from build123d import *

# Parameters (mm, degrees)
F3_DEPTH = 46.501
F5_D     = 14
F6_R     = 2
F7_R     = 1
F8_SIZE  = 1
F9_SIZE  = 0.5
F10_R    = 0.4


with BuildPart() as f1:
    # F0 (on Right) → F1 (revolve)
    with BuildSketch(Plane.YZ):
        Polygon((1.5, 26), (0, 26), (0, 16), (46.5, 16), (46.5, 28), (19.5, 28), (19.5, 62.5), (1.5, 62.5), align=None)
    revolve(axis=Axis((0, 26.823761, 0), (0, 1, 0)))

    # F2 (on face) → F3 (cut, through all)
    with BuildSketch(Plane(origin=(0, 46.5, 0), x_dir=(-1, 0, 0), z_dir=(0, 1, 0))):
        with BuildLine():
            ThreePointArc((4, 15.491933), (0, 16), (-4, 15.491933))
            Line((-4, 15.491933), (-4, 12))
            Line((-4, 12), (4, 12))
            Line((4, 12), (4, 15.491933))
        make_face()
        with BuildLine():
            Line((4, 18.4), (-4, 18.4))
            Line((-4, 18.4), (-4, 15.491933))
            ThreePointArc((-4, 15.491933), (0, 16), (4, 15.491933))
            Line((4, 15.491933), (4, 18.4))
        make_face()
    extrude(amount=-F3_DEPTH, mode=Mode.SUBTRACT)

    # F5 (through all)
    with Locations(Plane(origin=(0, 19.5, 0), x_dir=(-1, 0, 0), z_dir=(0, 1, 0))):
        with Locations((-30.052038, 30.052038), (30.052038, 30.052038), (-30.052038, -30.052038), (30.052038, -30.052038)):
            Hole(F5_D / 2)

    # F6
    f6_edges = [f1.edges().sort_by_distance(p)[0] for p in [
        (0, 19.5, -28),
        (0, 46.5, -28),
    ]]
    fillet(f6_edges, radius=F6_R)

    # F7
    f7_edges = [f1.edges().sort_by_distance(p)[0] for p in [
        (0, 19.5, -62.5),
    ]]
    fillet(f7_edges, radius=F7_R)

    # F8
    f8_edges = [f1.edges().sort_by_distance(p)[0] for p in [
        (0, 1.5, -62.5),
    ]]
    chamfer(f8_edges, length=F8_SIZE)

    # F9
    f9_edges = [f1.edges().sort_by_distance(p)[0] for p in [
        (0, 0, -26),
    ]]
    chamfer(f9_edges, length=F9_SIZE)

    # F10
    f10_edges = [f1.edges().sort_by_distance(p)[0] for p in [
        (0, 1.5, -26),
    ]]
    fillet(f10_edges, radius=F10_R)


solid = f1.part
Verification items for the finished model (mm, model axes). A direction names the side the tool comes from. Coordinates: 2 decimals unless noted, no trailing zeros. Order: outer loops, then holes, each group sorted by start corner. A loop starts at its lowest first (then second) coordinate and runs counter-clockwise, first axis right, second up.
Item 1: Section check C-C, the plane y = 26. Enter the section's corners in (x, z), then the cut area to 3 significant figures.
Filled in:
outline: circle Ø56 at (0, 0); hole (-4, 15.49) arc R16 ccw (long way) to (4, 15.49) - (4, 18.4) - (-4, 18.4) - close
area: 1,640 mm2
Item 2: Depth check by flat-ended pin: pin 1 (8 mm diameter, centred on x = 49, z = -20, fed in from +Y); pin 2 (22.5 mm diameter, centred on x = -30.05, z = 30.05, fed in from -Y); pin 3 (4 mm diameter, centred on x = -6.5, y = 41.5, fed in from +Z). Enter the tip coordinate at first touch or a pass-through.
Filled in:
pin 1: stops at y = 19.5
pin 2: stops at y = 1.5
pin 3: stops at z = 27.64
Item 3: Section check D-D, the plane y = 7. Enter the section's corners in (x, z), then the cut area to 3 significant figures.
Filled in:
outline: circle Ø125 at (0, 0); hole circle Ø14 at (-30.05, -30.05); hole circle Ø14 at (-30.05, 30.05); hole (-4, 15.49) arc R16 ccw (long way) to (4, 15.49) - (4, 18.4) - (-4, 18.4) - close; hole circle Ø14 at (30.05, -30.05); hole circle Ø14 at (30.05, 30.05)
area: 10,800 mm2
Item 4: Release check for a two-part mould opening along X. For faces 5 (the face through (12, 46.5, -11)), 6 (the face through (0.647, 23.576, -15.987)), 7 (the face through (2.75, 10.39, -62.44)), 8 (the face through (23.06, 10.37, -29.74)) record: +X half, -X half, draft (parallel to the pull), parting line (faces both ways), or undercut.
Filled in:
face 5: draft
face 6: undercut
face 7: parting line
face 8: undercut
Item 5: Access from +Z, -Z, +X, -X, +Y, -Y to the whole of each face (thin tool, end or side, straight path). Record for faces 1 (the face through (4, 24, 17)), 2 (the face through (-11, 0, -12)), 3 (the face through (-10.724, 32.839, 25.865)), 4 (the face through (-15.821, 0.796, -20.633)).
Filled in:
face 1: +Y, -Y
face 2: +Z, -Z, +X, -X, -Y
face 3: +Y
face 4: -Y
Item 6: Section check A-A, the plane x = 0. Enter the section's corners in (y, z).
Filled in:
outline: (0, -25.5) - (0.5, -26) - (1.1, -26) arc R0.4 cw to (1.5, -26.4) - (1.5, -61.5) - (2.5, -62.5) - (18.5, -62.5) arc R1 ccw to (19.5, -61.5) - (19.5, -30) arc R2 cw to (21.5, -28) - (44.5, -28) arc R2 ccw to (46.5, -26) - (46.5, -16) - (0, -16) - close; (0, 18.4) - (46.5, 18.4) - (46.5, 26) arc R2 ccw to (44.5, 28) - (21.5, 28) arc R2 cw to (19.5, 30) - (19.5, 61.5) arc R1 ccw to (18.5, 62.5) - (2.5, 62.5) - (1.5, 61.5) - (1.5, 26.4) arc R0.4 cw to (1.1, 26) - (0.5, 26) - (0, 25.5) - close
Item 7: Material ranges on L1, parallel to Y at x = -45.5, z = 19; L2, parallel to X at y = 32.5, z = 0; L3, parallel to X at y = 22.5, z = 13.5, recorded low to high.
Filled in:
L1: y = 1.5 to 19.5
L2: x = -28 to -16, 16 to 28
L3: x = -24.53 to -8.59, 8.59 to 24.53
Item 8: Section check B-B, the plane z = 0. Enter the section's corners in (x, y), then the cut area to 3 significant figures.
Filled in:
outline: (-62.5, 2.5) - (-61.5, 1.5) - (-26.4, 1.5) arc R0.4 cw to (-26, 1.1) - (-26, 0.5) - (-25.5, 0) - (-16, 0) - (-16, 46.5) - (-26, 46.5) arc R2 ccw to (-28, 44.5) - (-28, 21.5) arc R2 cw to (-30, 19.5) - (-61.5, 19.5) arc R1 ccw to (-62.5, 18.5) - close; (16, 0) - (25.5, 0) - (26, 0.5) - (26, 1.1) arc R0.4 cw to (26.4, 1.5) - (61.5, 1.5) - (62.5, 2.5) - (62.5, 18.5) arc R1 ccw to (61.5, 19.5) - (30, 19.5) arc R2 cw to (28, 21.5) - (28, 44.5) arc R2 ccw to (26, 46.5) - (16, 46.5) - close
area: 2,350 mm2
